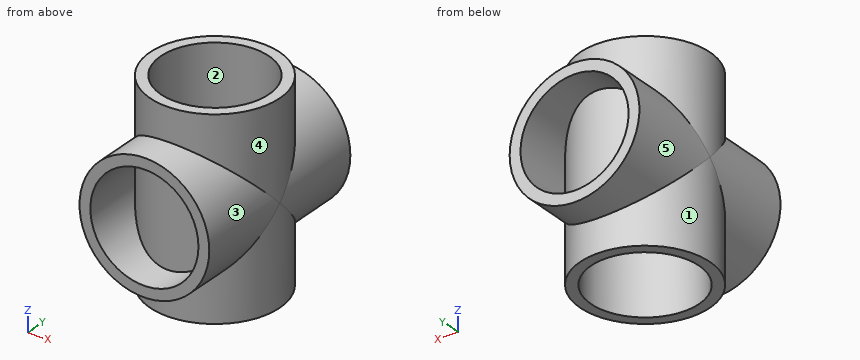
from build123d import *

# Parameters (mm, degrees)
SKETCH1_R                = 6
SKETCH1_R_2              = 5
BOSS_EXTRUDE1_DEPTH      = 9
BOSS_EXTRUDE1_DEPTH_BACK = 9
SKETCH2_R                = 6
BOSS_EXTRUDE2_DEPTH      = 9
BOSS_EXTRUDE2_DEPTH_BACK = 9
SKETCH3_R                = 5
CUT_EXTRUDE1_DEPTH       = 19


with BuildPart() as part:
    # Sketch1 → Boss-Extrude1 (new body, two sides)
    with BuildSketch(Plane(origin=(0, 0, 0), x_dir=(1, 0, 0), z_dir=(0, 1, 0))) as boss_extrude1_sk:
        Circle(SKETCH1_R)
        Circle(SKETCH1_R_2, mode=Mode.SUBTRACT)
    extrude(amount=BOSS_EXTRUDE1_DEPTH)
    extrude(boss_extrude1_sk.sketch, amount=-BOSS_EXTRUDE1_DEPTH_BACK)

    # Sketch2 → Boss-Extrude2 (add, two sides)
    with BuildSketch(Plane.XY) as boss_extrude2_sk:
        Circle(SKETCH2_R)
    extrude(amount=BOSS_EXTRUDE2_DEPTH)
    extrude(boss_extrude2_sk.sketch, amount=-BOSS_EXTRUDE2_DEPTH_BACK)

    # Sketch3 → Cut-Extrude1 (cut, through all)
    with BuildSketch(Plane(origin=(0, 0, -9), x_dir=(-1, 0, 0), z_dir=(0, 0, -1))):
        Circle(SKETCH3_R)
    extrude(amount=-CUT_EXTRUDE1_DEPTH, mode=Mode.SUBTRACT)


solid = part.part
Geometry check sheet. Reference: the model listing, model coordinates, mm. Face numbers are marked on the shaded views. A direction names the side the tool comes from. Round coordinates to 2 decimals unless told otherwise and drop trailing zeros. Loops run counter-clockwise (first coordinate to the right, second up) from the corner with the lowest first, then second, coordinate; pieces in that order, holes last. Notation, with made-up numbers: (73.25, 35) - (103.25, 35) arc R18 cw to (103.25, 63) - close; hole circle Ø11 at (-12, 64.25). An arc over 180 degrees is marked (long way). One line per question, with ' | ' between items. Start each with the question number.
1. Cross-section at A-A on x = 0. Record the cut outline in (y, z), then the cut area to 3 significant figures.
2. Depth check by flat-ended pin: pin 1 (1 mm diameter, centred on y = 3.5, z = 2.5, fed in from -X); pin 2 (5 mm diameter, centred on x = -2, z = 0.5, fed in from -Y); pin 3 (6 mm diameter, centred on x = 0, z = 0, fed in from +Y). Enter the tip coordinate at first touch or a pass-through.
3. Cross-section at B-B on y = -2.75. Record the cut outline in (x, z), then the cut area to 3 significant figures.
4. Draft check along Y on the marked faces 1 and 2. Enter one of: released by +Y, released by -Y, zero draft, split by the parting line, or undercut.
5. Cross-section at C-C on z = 4.5. Record the cut outline in (x, y), then the cut area to 3 significant figures.
6. Scan line: line 1 (Z direction, x = 0, y = -6.5). Record every from-to range of solid material in increasing order. Write a range as [from, to].
7. Cross-section at D-D on y = 4.5. Record the cut outline in (x, z).
8. Tool access check on the marked faces 3, 4 and 5. Record the directions out of +Z, -Z, +X, -X, +Y, -Y that give a thin tool (end or side, any length) a straight path to the whole face; none if there is none.
Taken from the geometry:
1) outline: (-9, -6) - (-6, -6) - (-6, -9) - (-5, -9) - (-5, 9) - (-6, 9) - (-6, 6) - (-9, 6) - (-9, 5) - (-6, 5) - (-6, -5) - (-9, -5) - close; (5, -9) - (6, -9) - (6, -6) - (9, -6) - (9, -5) - (6, -5) - (6, 5) - (9, 5) - (9, 6) - (6, 6) - (6, 9) - (5, 9) - close | area: 48.0 mm²
2) pin 1: x = -5.66 | pin 2: y = -6 | pin 3: y = 6
3) outline: (-5.33, -9) - (-4.18, -9) - (-4.18, 9) - (-5.33, 9) - (-5.33, 2.75) arc R6 ccw to (-5.33, -2.75) - close; (4.18, -9) - (5.33, -9) - (5.33, -2.75) arc R6 ccw to (5.33, 2.75) - (5.33, 9) - (4.18, 9) - close | area: 46.6 mm²
4) face 1: split by the parting line | face 2: undercut
5) outline: (-3.97, -9) - (-2.18, -9) - (-2.18, -5.59) arc R6 ccw to (2.18, -5.59) - (2.18, -9) - (3.97, -9) - (3.97, -4.5) arc R6 ccw to (3.97, 4.5) - (3.97, 9) - (2.18, 9) - (2.18, 5.59) arc R6 ccw to (-2.18, 5.59) - (-2.18, 9) - (-3.97, 9) - (-3.97, 4.5) arc R6 ccw to (-3.97, -4.5) - close; hole circle Ø10 at (0, 0) | area: 62.3 mm²
6) line 1: [-6, -5], [5, 6]
7) outline: (-3.97, -9) - (-2.18, -9) - (-2.18, 9) - (-3.97, 9) - (-3.97, 4.5) arc R6 ccw to (-3.97, -4.5) - close; (2.18, -9) - (3.97, -9) - (3.97, -4.5) arc R6 ccw to (3.97, 4.5) - (3.97, 9) - (2.18, 9) - close; hole (-3.97, -3.04) - (-3.97, 3.04) arc R5 ccw to start; hole (3.97, -3.04) arc R5 ccw to (3.97, 3.04) - close
8) face 3: -Y | face 4: +Z | face 5: +Y
